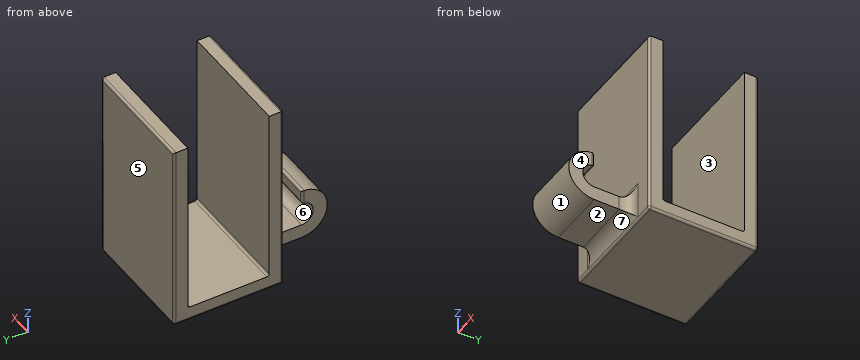
```python
from build123d import *

# Parameters (mm, degrees)
BOSS_EXTRUDE1_DEPTH = 25.4
BOSS_EXTRUDE3_DEPTH = 25.4
CUT_EXTRUDE5_DEPTH  = 6.35
CUT_EXTRUDE6_START  = -6.35
CUT_EXTRUDE6_DEPTH  = 6.35
FILLET1_R           = 2.5
FILLET2_R           = 2.5
FILLET3_R           = 0.5
FILLET4_R           = 0.5
FILLET5_R           = 0.5


with BuildPart() as part:
    # Sketch1 → Boss-Extrude1 (new body)
    with BuildSketch(Plane(origin=(0, 0, 0), x_dir=(0, 0, -1), z_dir=(1, 0, 0))):
        Polygon((0, 0), (38.1, 0), (38.1, -17.5), (0, -17.5), (1.83e-15, -20.500000000000007), (41.1, -20.500000000000007), (41.099999999999994, 3), (-1.8e-16, 2.999999999999995), align=None)
    extrude(amount=BOSS_EXTRUDE1_DEPTH)

    # Sketch7 → Boss-Extrude3 (add)
    with BuildSketch(Plane.ZY):
        with BuildLine():
            Line((-38.1, -20.500000000000007), (-38.10000000000001, -28.33631785905126))
            ThreePointArc((-38.10000000000001, -28.33631785905126), (-32.6, -33.83631785905126), (-27.100000000000005, -28.336317859051263))
            Line((-27.100000000000005, -28.336317859051263), (-30.100000000000005, -28.33631785905126))
            ThreePointArc((-30.100000000000005, -28.33631785905126), (-32.607239712312804, -30.821806864386282), (-35.1, -28.32179632065465))
            Line((-35.1, -28.32179632065465), (-35.1, -20.500000000000007))
            Line((-35.1, -20.500000000000007), (-38.1, -20.500000000000007))
        make_face()
    extrude(amount=-BOSS_EXTRUDE3_DEPTH)

    # Sketch8 → Cut-Extrude5 (cut)
    with BuildSketch(Plane.ZY):
        with BuildLine():
            Line((-35.1, -20.500000000000007), (-38.1, -20.500000000000007))
            Line((-38.1, -20.500000000000007), (-38.10000000000001, -28.3363178590513))
            ThreePointArc((-38.10000000000001, -28.3363178590513), (-32.59999999999998, -33.83631785905126), (-27.100000000000005, -28.336317859051263))
            Line((-27.100000000000005, -28.336317859051263), (-30.10000000000001, -28.33631785905126))
            ThreePointArc((-30.10000000000001, -28.33631785905126), (-32.6072397123128, -30.82180686438628), (-35.1, -28.321796320654666))
            Line((-35.1, -28.321796320654666), (-35.1, -20.500000000000007))
        make_face()
    extrude(amount=-CUT_EXTRUDE5_DEPTH, mode=Mode.SUBTRACT)

    # Sketch9 → Cut-Extrude6 (cut)
    with BuildSketch(Plane(origin=(25.4, 0, 0), x_dir=(0, 0, -1), z_dir=(1, 0, 0)).offset(CUT_EXTRUDE6_START)):
        with BuildLine():
            Line((35.1, -20.500000000000007), (38.1, -20.500000000000007))
            Line((38.1, -20.500000000000007), (38.10000000000001, -28.33631785905126))
            ThreePointArc((38.10000000000001, -28.33631785905126), (32.6, -33.83631785905126), (27.100000000000005, -28.336317859051263))
            Line((27.100000000000005, -28.336317859051263), (30.10000000000001, -28.33631785905126))
            ThreePointArc((30.10000000000001, -28.33631785905126), (32.607239712312804, -30.82180686438628), (35.1, -28.32179632065465))
            Line((35.1, -28.32179632065465), (35.1, -20.500000000000007))
        make_face()
    extrude(amount=CUT_EXTRUDE6_DEPTH, mode=Mode.SUBTRACT)

    # Fillet1
    fillet1_edges = [part.edges().sort_by_distance(p)[0] for p in [
        (12.7, -20.500000000000007, -35.1),
        (12.7, -20.500000000000007, -38.1),
    ]]
    fillet(fillet1_edges, radius=FILLET1_R)

    # Fillet2
    fillet2_edges = [part.edges().sort_by_distance(p)[0] for p in [
        (6.35, -20.500000000000007, -36.599999999999994),
        (19.049999999999997, -20.500000000000007, -36.599999999999994),
    ]]
    fillet(fillet2_edges, radius=FILLET2_R)

    # Fillet3
    fillet3_edges = [part.edges().sort_by_distance(p)[0] for p in [
        (12.7, 2.999999999999995, 1.8e-16),
        (12.7, 3, -41.099999999999994),
        (12.7, -20.500000000000007, -41.1),
        (12.7, -20.500000000000007, -1.83e-15),
        (25.4, -20.500000000000007, -20.550000000000004),
        (25.4, -8.750000000000004, -41.099999999999994),
        (25.4, 2.9999999999999973, -20.549999999999997),
        (0, 2.9999999999999973, -20.549999999999997),
        (0, -8.750000000000004, -41.099999999999994),
        (0, -20.500000000000007, -20.55),
    ]]
    fillet(fillet3_edges, radius=FILLET3_R)

    # Fillet4
    fillet4_edges = [part.edges().sort_by_distance(p)[0] for p in [
        (6.35, -28.336317859051263, -28.60000000000001),
        (12.7, -28.336317859051263, -27.100000000000005),
        (12.7, -28.33631785905126, -30.100000000000005),
        (19.049999999999997, -28.336317859051263, -28.60000000000001),
    ]]
    fillet(fillet4_edges, radius=FILLET4_R)

    # Fillet5
    fillet5_edges = [part.edges().sort_by_distance(p)[0] for p in [
        (12.7, -17.5, -38.1),
        (12.7, 0, -38.1),
    ]]
    fillet(fillet5_edges, radius=FILLET5_R)


solid = part.part
```
Verification items for the finished model (mm, model axes). Face numbers are marked on the shaded views. A direction names the side the tool comes from. Round coordinates to 2 decimals unless told otherwise and drop trailing zeros. Write each loop counter-clockwise with the first axis right and the second up, starting at its lowest first coordinate (ties: lowest second). Pieces come first, ordered by that corner, then holes. Notation, with made-up numbers: (-26, -36) - (-7, -36) arc R27 cw to (-7, -12) - close; hole circle Ø2 at (22, -9). An arc over 180 degrees is marked (long way). Answer as a JSON object with one key per item and string values. Group by question number.
Q1. Section check D-D, the plane z = -37. Enter the section's corners in (x, y).
Q2. Section check A-A, the plane z = -10.5. Enter the section's corners in (x, y), plus the area to 3 significant figures.
Q3. Go/stop test with flat-tipped pins: pin 1 Ø1.6 at (x, y) = (13, -25) entering from +Z; pin 2 Ø12 at (y, z) = (-9, -24.5) entering from -X (1 decimal); pin 3 Ø1.6 at (x, y) = (11.5, -24.5) entering from -Z; pin 4 Ø8.5 at (y, z) = (-29.5, -33.5) entering from -X. Record where each tip stops, or that it passes through.
Q4. Mould release check, pull along Y, two halves, no side actions. Record for the marked faces 5, 6 and 7: released by +Y, released by -Y, zero draft, split by the parting line, or undercut.
Q5. Thickness scan on line 1 (Y direction, x = 24, z = -10); line 2 (Y direction, x = 19.75, z = -33.5); line 3 (Z direction, x = 2, y = -5). Record the ranges inside material, lowest first.
Q6. Section check C-C, the plane y = -3. Enter the section's corners in (x, z).
Q7. Tool access check on the marked faces 1, 2, 3 and 4. Record the directions out of +Z, -Z, +X, -X, +Y, -Y that give a thin tool (end or side, any length) a straight path to the whole face; none if there is none.
Q8. Section check B-B, the plane x = 9.5. Enter the section's corners in (y, z).
Found:
{
 "1": {"outline": "(0, -20) arc R0.5 ccw to (0.5, -20.5) - (3.85, -20.5) arc R2.5 cw to (6.35, -23) - (6.35, -31.64) - (19.05, -31.64) - (19.05, -23) arc R2.5 cw to (21.55, -20.5) - (24.9, -20.5) arc R0.5 ccw to (25.4, -20) - (25.4, -17.5) - (0, -17.5) - close; (0, 0) - (25.4, 0) - (25.4, 2.5) arc R0.5 ccw to (24.9, 3) - (0.5, 3) arc R0.5 ccw to (0, 2.5) - close"},
 "2": {"outline": "(0, -20) arc R0.5 ccw to (0.5, -20.5) - (24.9, -20.5) arc R0.5 ccw to (25.4, -20) - (25.4, -17.5) - (0, -17.5) - close; (0, 0) - (25.4, 0) - (25.4, 2.5) arc R0.5 ccw to (24.9, 3) - (0.5, 3) arc R0.5 ccw to (0, 2.5) - close", "area": "152 mm^2"},
 "3": {"pin 1": "stops at z = -35.1", "pin 2": "passes through", "pin 3": "stops at z = -38.1", "pin 4": "stops at x = 6.35"},
 "4": {"face 5": "released by +Y", "face 6": "undercut", "face 7": "released by -Y"},
 "5": {"line 1": "y = -20.5 to -17.5, 0 to 3", "line 2": "y = -20.67 to -17.5, 0 to 3", "line 3": "z = -41.1 to -38.1"},
 "6": {"outline": "(0, -40.6) arc R0.5 ccw to (0.5, -41.1) - (24.9, -41.1) arc R0.5 ccw to (25.4, -40.6) - (25.4, -38.1) - (0, -38.1) - close"},
 "7": {"face 1": "+X, -X, -Y", "face 2": "-Z, +X, -X, -Y", "face 3": "+Z, +X, -X", "face 4": "+Z, -Z, +X, -Y"},
 "8": {"outline": "(-28.89, -27.13) arc R5.5 ccw to (-28.34, -38.1) - (-23, -38.1) arc R2.5 cw to (-20.5, -40.6) arc R0.5 ccw to (-20, -41.1) - (2.5, -41.1) arc R0.5 ccw to (3, -40.6) - (3, -0.5) arc R0.5 ccw to (2.5, 0) - (0, 0) - (0, -37.6) arc R0.5 cw to (-0.5, -38.1) - (-17, -38.1) arc R0.5 cw to (-17.5, -37.6) - (-17.5, 0) - (-20, 0) arc R0.5 ccw to (-20.5, -0.5) - (-20.5, -32.6) arc R2.5 cw to (-23, -35.1) - (-28.32, -35.1) arc R2.5 cw to (-28.75, -30.14) arc R0.5 ccw to (-28.34, -29.64) - (-28.34, -27.63) arc R0.5 ccw to start"}
}
